Input: part model. Units: mm. Frame: model coordinates. A direction names the side the tool comes from. Give positions to 0.01 mm unless a question says otherwise; leave off trailing zeros. Write each loop counter-clockwise with the first axis right and the second up, starting at its lowest first coordinate (ties: lowest second). Pieces come first, ordered by that corner, then holes.
```python
from build123d import *

# Parameters (mm, degrees)
F0_W     = 76.2
F0_H     = 50.8
F0_R     = 12.7
F1_DEPTH = 12.7
F2_W     = 6.35
F2_H     = 50.8
F3_DEPTH = 2.54
F5_DEPTH = 50.801
F6_R     = 4.7625
F7_DEPTH = 12.7


with BuildPart() as f1:
    # F0 (on Top) → F1 (new body)
    with BuildSketch(Plane.XY):
        with Locations((0.796007, 0.286434)):
            Rectangle(F0_W, F0_H)
        Circle(F0_R, mode=Mode.SUBTRACT)
    extrude(amount=F1_DEPTH)

    # F2 (on face) → F3 (cut)
    with BuildSketch(Plane.XY.offset(12.7)):
        with Locations((-31.588993, 0.286434)):
            Rectangle(F2_W, F2_H)
        with BuildLine():
            Line((-5.894164, -11.249392), (-5.894164, -25.113566))
            Line((-5.894164, -25.113566), (4.265836, -25.113566))
            Line((4.265836, -25.113566), (4.265836, -11.962134))
            ThreePointArc((4.265836, -11.962134), (-0.888743, -12.668865), (-5.894164, -11.249392))
        make_face()
        with BuildLine():
            Line((4.265836, 25.686434), (-5.894164, 25.686434))
            Line((-5.894164, 25.686434), (-5.894164, 11.249392))
            ThreePointArc((-5.894164, 11.249392), (-0.888743, 12.668865), (4.265836, 11.962134))
            Line((4.265836, 11.962134), (4.265836, 25.686434))
        make_face()
    extrude(amount=-F3_DEPTH, mode=Mode.SUBTRACT)

    # F4 (on face) → F5 (cut, through all)
    with BuildSketch(Plane.XZ.offset(25.113566)):
        Polygon((30.935836, 12.7), (18.235836, 12.7), (15.302896, 7.62), (33.868775, 7.62), align=None)
    extrude(amount=-F5_DEPTH, mode=Mode.SUBTRACT)

    # F6 (on face) → F7 (join)
    with BuildSketch(Plane.YZ.offset(38.896007)):
        with Locations((0, 6.35)):
            Circle(F6_R)
    extrude(amount=F7_DEPTH)


solid = f1.part
```
Q1. Pin query (flat end, axial travel): pin 1 (9.5 mm diameter, centred on x = 25, y = 3, fed in from +Z); pin 2 (11 mm diameter, centred on x = 0, y = 18.5, fed in from +Z); pin 3 (0.8 mm diameter, centred on y = 11.5, z = 11, fed in from +X); pin 4 (3 mm diameter, centred on x = -30.5, y = 4.5, fed in from +Z). Return the tip coordinate at first contact, or that it passes through.
Q2. Section A-A, the plane y = 0. Return the cut outline in (x, z).
Q3. Section D-D, the plane y = 17.5. Return the cut outline in (x, z).
Q4. Material intervals for line 1 along Y through (x, z) = (0, 3.5); line 2 along X through (y, z) = (-12, 11.5); line 3 along X through (y, z) = (0, 8.75), sorted ascending.
Q5. Mould query, pull axis X, two halves, no side actions, for faces 1 (the flat face through (-36, 1, 12.7)), 2 (the flat face through (-37.304, 0, 6)), 3 (the flat face through (16.79, -0.069, 10.196)). Classes: +X half, -X half, draft (parallel to the pull), parting line (faces both ways), or undercut.
Q6. Access query for faces 4 (the flat face through (35, 1, 12.7)), 5 (the flat face through (-32, 1, 10.16)), 6 (the flat face through (24, 0, 7.62)). Directions: +Z, -Z, +X, -X, +Y, -Y. A direction counts if a zero-diameter tool reaches every point of the face in a straight line with its end or side. Return the directions, or none.
Q7. Section B-B, the plane z = 6.35. Return the cut outline in (x, y), then the cut area to 3 significant figures.
Q8. Section C-C, the plane x = 0. Return the cut outline in (y, z), then the cut area to 3 significant figures.
Solutions:
1. pin 1: stops at z = 7.62
1. pin 2: stops at z = 12.7
1. pin 3: stops at x = 38.9
1. pin 4: stops at z = 10.16
2. outline: (-37.3, 0) - (-12.7, 0) - (-12.7, 12.7) - (-28.41, 12.7) - (-28.41, 10.16) - (-34.76, 10.16) - (-34.76, 12.7) - (-37.3, 12.7) - close; (12.7, 0) - (38.9, 0) - (38.9, 1.59) - (51.6, 1.59) - (51.6, 11.11) - (38.9, 11.11) - (38.9, 12.7) - (30.94, 12.7) - (33.87, 7.62) - (15.3, 7.62) - (18.24, 12.7) - (12.7, 12.7) - close
3. outline: (-37.3, 0) - (38.9, 0) - (38.9, 12.7) - (30.94, 12.7) - (33.87, 7.62) - (15.3, 7.62) - (18.24, 12.7) - (4.27, 12.7) - (4.27, 10.16) - (-5.89, 10.16) - (-5.89, 12.7) - (-28.41, 12.7) - (-28.41, 10.16) - (-34.76, 10.16) - (-34.76, 12.7) - (-37.3, 12.7) - close
4. line 1: y = -25.11 to -12.7, 12.7 to 25.69
4. line 2: x = -37.3 to -34.76, -28.41 to -5.89, 4.27 to 17.54, 31.63 to 38.9
4. line 3: x = -37.3 to -12.7, 12.7 to 15.96, 33.22 to 51.6
5. face 1: draft
5. face 2: -X half
5. face 3: undercut
6. face 4: +Z, +X, -X, +Y, -Y
6. face 5: +Z, +Y, -Y
6. face 6: +Y, -Y
7. outline: (-37.3, -25.11) - (38.9, -25.11) - (38.9, -4.76) - (51.6, -4.76) - (51.6, 4.76) - (38.9, 4.76) - (38.9, 25.69) - (-37.3, 25.69) - close; hole circle Ø25.4 at (0, 0)
7. area: 3,490 mm2
8. outline: (-25.11, 0) - (-12.7, 0) - (-12.7, 10.16) - (-25.11, 10.16) - close; (12.7, 0) - (25.69, 0) - (25.69, 10.16) - (12.7, 10.16) - close
8. area: 258 mm2
